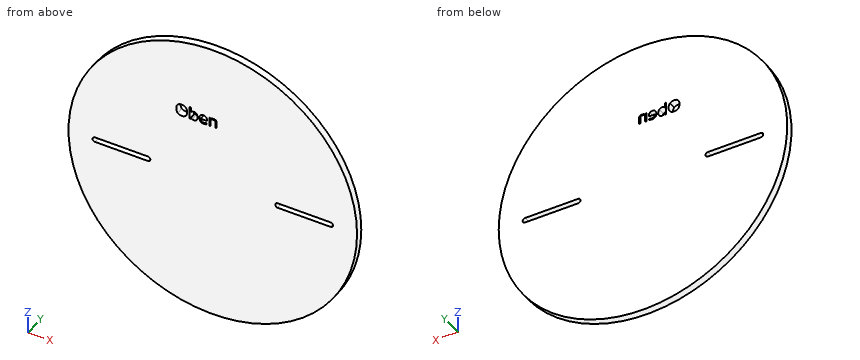
from build123d import *

# Parameters (mm, degrees)
F0_R     = 300.0001975894
F1_DEPTH = 15


with BuildPart() as f1:
    # F0 (on Front) → F1 (new body)
    with BuildSketch(Plane.XZ):
        Circle(F0_R)
        with BuildLine():
            ThreePointArc((-245.0001975894, -5.1), (-250.1001975894, 0), (-245.0001975894, 5.1))
            Line((-245.0001975894, 5.1), (-135, 5.1))
            ThreePointArc((-135, 5.1), (-129.9, 0), (-135, -5.1))
            Line((-135, -5.1), (-245.0001975894, -5.1))
        make_face(mode=Mode.SUBTRACT)
        with BuildLine():
            ThreePointArc((135.0291466713, -5.1012321273), (129.9, -0.0303787986), (134.9708533287, 5.0987678727))
            Line((134.9708533287, 5.0987678727), (245.0001975894, 5.0987678727))
            ThreePointArc((245.0001975894, 5.0987678727), (250.1001975894, -0.0012321273), (245.0001975894, -5.1012321273))
            Line((245.0001975894, -5.1012321273), (135.0291466713, -5.1012321273))
        make_face(mode=Mode.SUBTRACT)
        with BuildLine():
            add(Edge.make_bspline(
                [(-56.2059473305, 147.280047389), (-53.2054559961, 143.8888953384), (-53.2054559961, 137.9204677295)],
                knots=[0, 0, 0, 1, 1, 1], degree=2))
            add(Edge.make_bspline(
                [(-53.2054559961, 137.9204677295), (-53.2054559961, 131.9683176504), (-56.216799017, 128.5581751484)],
                knots=[0, 0, 0, 1, 1, 1], degree=2))
            add(Edge.make_bspline(
                [(-56.216799017, 128.5581751484), (-59.2281420379, 125.1480326464), (-64.5834493561, 125.1480326464)],
                knots=[0, 0, 0, 1, 1, 1], degree=2))
            add(Edge.make_bspline(
                [(-64.5834493561, 125.1480326464), (-70.0581252264, 125.1480326464), (-73.034200266, 128.4984908723)],
                knots=[0, 0, 0, 1, 1, 1], degree=2))
            add(Edge.make_bspline(
                [(-73.034200266, 128.4984908723), (-76.0102753055, 131.8489490982), (-76.0102753055, 137.9530227892)],
                knots=[0, 0, 0, 1, 1, 1], degree=2))
            add(Edge.make_bspline(
                [(-76.0102753055, 137.9530227892), (-76.0102753055, 144.0082638906), (-73.0260615011, 147.339731665)],
                knots=[0, 0, 0, 1, 1, 1], degree=2))
            add(Edge.make_bspline(
                [(-73.0260615011, 147.339731665), (-70.0418476966, 150.6711994395), (-64.5508942964, 150.6711994395)],
                knots=[0, 0, 0, 1, 1, 1], degree=2))
            add(Edge.make_bspline(
                [(-64.5508942964, 150.6711994395), (-59.2064386648, 150.6711994395), (-56.2059473305, 147.280047389)],
                knots=[0, 0, 0, 1, 1, 1], degree=2))
        make_face(mode=Mode.SUBTRACT)
        with BuildLine():
            add(Edge.make_bspline(
                [(-45.2891506494, 141.5991894739), (-43.3249953817, 144.3772212337), (-39.4563691225, 144.3772212337)],
                knots=[0, 0, 0, 1, 1, 1], degree=2))
            add(Edge.make_bspline(
                [(-39.4563691225, 144.3772212337), (-35.7939249079, 144.3772212337), (-33.7673724425, 141.8759074812)],
                knots=[0, 0, 0, 1, 1, 1], degree=2))
            add(Edge.make_bspline(
                [(-33.7673724425, 141.8759074812), (-31.7408199771, 139.3745937288), (-31.7408199771, 134.800607843)],
                knots=[0, 0, 0, 1, 1, 1], degree=2))
            add(Edge.make_bspline(
                [(-31.7408199771, 134.800607843), (-31.7408199771, 130.221196114), (-33.7836499724, 127.6846143802)],
                knots=[0, 0, 0, 1, 1, 1], degree=2))
            add(Edge.make_bspline(
                [(-33.7836499724, 127.6846143802), (-35.8264799676, 125.1480326464), (-39.4563691225, 125.1480326464)],
                knots=[0, 0, 0, 1, 1, 1], degree=2))
            add(Edge.make_bspline(
                [(-39.4563691225, 125.1480326464), (-41.2740266216, 125.1480326464), (-42.7742722887, 125.8181242916)],
                knots=[0, 0, 0, 1, 1, 1], degree=2))
            add(Edge.make_bspline(
                [(-42.7742722887, 125.8181242916), (-44.2745179559, 126.4882159368), (-45.2891506494, 127.8826576599)],
                knots=[0, 0, 0, 1, 1, 1], degree=2))
            Line((-45.2891506494, 127.8826576599), (-45.4953326941, 127.8826576599))
            Line((-45.4953326941, 127.8826576599), (-46.0867496117, 125.4898607731))
            Line((-46.0867496117, 125.4898607731), (-48.1051633122, 125.4898607731))
            Line((-48.1051633122, 125.4898607731), (-48.1051633122, 151.8757366478))
            Line((-48.1051633122, 151.8757366478), (-45.2891506494, 151.8757366478))
            Line((-45.2891506494, 151.8757366478), (-45.2891506494, 145.4623898899))
            add(Edge.make_bspline(
                [(-45.2891506494, 145.4623898899), (-45.2891506494, 143.3083301074), (-45.4247967314, 141.5991894739)],
                knots=[0, 0, 0, 1, 1, 1], degree=2))
            Line((-45.4247967314, 141.5991894739), (-45.2891506494, 141.5991894739))
        make_face(mode=Mode.SUBTRACT)
        with BuildLine():
            add(Edge.make_bspline(
                [(-15.761711515, 125.430176497), (-17.0910431189, 125.1480326464), (-18.9738107373, 125.1480326464)],
                knots=[0, 0, 0, 1, 1, 1], degree=2))
            add(Edge.make_bspline(
                [(-18.9738107373, 125.1480326464), (-23.0920257875, 125.1480326464), (-25.4766839094, 127.6601980854)],
                knots=[0, 0, 0, 1, 1, 1], degree=2))
            add(Edge.make_bspline(
                [(-25.4766839094, 127.6601980854), (-27.8613420313, 130.1723635245), (-27.8613420313, 134.626980858)],
                knots=[0, 0, 0, 1, 1, 1], degree=2))
            add(Edge.make_bspline(
                [(-27.8613420313, 134.626980858), (-27.8613420313, 139.1250049378), (-25.6475979727, 141.7701035373)],
                knots=[0, 0, 0, 1, 1, 1], degree=2))
            add(Edge.make_bspline(
                [(-25.6475979727, 141.7701035373), (-23.4338539142, 144.4152021367), (-19.7008737369, 144.4152021367)],
                knots=[0, 0, 0, 1, 1, 1], degree=2))
            add(Edge.make_bspline(
                [(-19.7008737369, 144.4152021367), (-16.2120565074, 144.4152021367), (-14.177365277, 142.1173575072)],
                knots=[0, 0, 0, 1, 1, 1], degree=2))
            add(Edge.make_bspline(
                [(-14.177365277, 142.1173575072), (-12.1426740467, 139.8195128778), (-12.1426740467, 136.0539776409)],
                knots=[0, 0, 0, 1, 1, 1], degree=2))
            Line((-12.1426740467, 136.0539776409), (-12.1426740467, 134.2743010448))
            Line((-12.1426740467, 134.2743010448), (-24.9422383462, 134.2743010448))
            add(Edge.make_bspline(
                [(-24.9422383462, 134.2743010448), (-24.8554248537, 131.0025175464), (-23.2873561456, 129.3069415212)],
                knots=[0, 0, 0, 1, 1, 1], degree=2))
            add(Edge.make_bspline(
                [(-23.2873561456, 129.3069415212), (-21.7192874374, 127.6113654959), (-18.870719715, 127.6113654959)],
                knots=[0, 0, 0, 1, 1, 1], degree=2))
            add(Edge.make_bspline(
                [(-18.870719715, 127.6113654959), (-15.8702283807, 127.6113654959), (-12.940273009, 128.8647352938)],
                knots=[0, 0, 0, 1, 1, 1], degree=2))
            Line((-12.940273009, 128.8647352938), (-12.940273009, 126.3525698547))
            add(Edge.make_bspline(
                [(-12.940273009, 126.3525698547), (-14.4323799112, 125.7123203476), (-15.761711515, 125.430176497)],
                knots=[0, 0, 0, 1, 1, 1], degree=2))
        make_face(mode=Mode.SUBTRACT)
        with BuildLine():
            Line((8.1933865699, 125.4898607731), (5.3773739071, 125.4898607731))
            Line((5.3773739071, 125.4898607731), (5.3773739071, 137.5135294834))
            add(Edge.make_bspline(
                [(5.3773739071, 137.5135294834), (5.3773739071, 139.7815319748), (4.3437507621, 140.9019686123)],
                knots=[0, 0, 0, 1, 1, 1], degree=2))
            add(Edge.make_bspline(
                [(4.3437507621, 140.9019686123), (3.3101276171, 142.0224052498), (1.1018094018, 142.0224052498)],
                knots=[0, 0, 0, 1, 1, 1], degree=2))
            add(Edge.make_bspline(
                [(1.1018094018, 142.0224052498), (-1.81186844, 142.0224052498), (-3.1683292602, 140.4461977767)],
                knots=[0, 0, 0, 1, 1, 1], degree=2))
            add(Edge.make_bspline(
                [(-3.1683292602, 140.4461977767), (-4.5247900804, 138.8699903036), (-4.5247900804, 135.2401011488)],
                knots=[0, 0, 0, 1, 1, 1], degree=2))
            Line((-4.5247900804, 135.2401011488), (-4.5247900804, 125.4898607731))
            Line((-4.5247900804, 125.4898607731), (-7.3408027432, 125.4898607731))
            Line((-7.3408027432, 125.4898607731), (-7.3408027432, 144.07337401))
            Line((-7.3408027432, 144.07337401), (-5.0510968787, 144.07337401))
            Line((-5.0510968787, 144.07337401), (-4.5953260431, 141.5286535113))
            Line((-4.5953260431, 141.5286535113), (-4.459679961, 141.5286535113))
            add(Edge.make_bspline(
                [(-4.459679961, 141.5286535113), (-3.5915450361, 142.9013918613), (-2.0316150929, 143.658296999)],
                knots=[0, 0, 0, 1, 1, 1], degree=2))
            add(Edge.make_bspline(
                [(-2.0316150929, 143.658296999), (-0.4716851496, 144.4152021367), (1.4436375285, 144.4152021367)],
                knots=[0, 0, 0, 1, 1, 1], degree=2))
            add(Edge.make_bspline(
                [(1.4436375285, 144.4152021367), (4.8022345194, 144.4152021367), (6.4978105446, 142.7955879173)],
                knots=[0, 0, 0, 1, 1, 1], degree=2))
            add(Edge.make_bspline(
                [(6.4978105446, 142.7955879173), (8.1933865699, 141.175973698), (8.1933865699, 137.6111946625)],
                knots=[0, 0, 0, 1, 1, 1], degree=2))
            Line((8.1933865699, 137.6111946625), (8.1933865699, 125.4898607731))
        make_face(mode=Mode.SUBTRACT)
    extrude(amount=F1_DEPTH)


solid = f1.part
The model under review builds one solid part; all positions refer to its coordinate system, in mm. Round coordinates to 2 decimals unless told otherwise and drop trailing zeros. Loops run counter-clockwise (first coordinate to the right, second up) from the corner with the lowest first, then second, coordinate; pieces in that order, holes last. Notation, with made-up numbers: M -14,66.5 L 6,66.5 A28 ccw 6,95.5 Z; hole C 62,-4 d6. An arc over 180 degrees is marked long. Answer as a JSON object with one key per item and string values.
Item 1: We need section C-C, the plane z = -175. State the section outline as (x, y) points.
Check sheet entries:
{"outline": "M -243.67,-15 L 243.67,-15 L 243.67,0 L -243.67,0 Z"}
Item 2: We need section D-D, the plane x = -192. State the section outline as (y, z) points.
Check sheet entries:
{"outline": "M -15,-230.51 L 0,-230.51 L 0,-5.1 L -15,-5.1 Z; M -15,5.1 L 0,5.1 L 0,230.51 L -15,230.51 Z"}
Item 3: We need section B-B, the plane y = -3.5. State how many separate pieces and enclosed holes the cut face has, and give its area (3 significant figures).
Check sheet entries:
{"separate pieces": "1", "enclosed holes": "6", "area": "279,000 mm2"}
Item 4: We need section A-A, the plane x = 169. State the section outline as (y, z) points, and give its area (3 significant figures).
Check sheet entries:
{"outline": "M -15,-247.87 L 0,-247.87 L 0,-5.1 L -15,-5.1 Z; M -15,5.1 L 0,5.1 L 0,247.87 L -15,247.87 Z", "area": "7,280 mm2"}
Item 5: Clearance check with flat-ended pins moving along their axes: P1, Ø1.4, axis at x = -6, y = -4, coming from the +Z side; P2, Ø1, axis at x = -128, y = -13, coming from the +Z side; P3, Ø2.5, axis at x = -46, y = -5.5, coming from the -Z side. State where each tip first meets the part, or that it passes through.
Check sheet entries:
{"P1": "z = 299.95", "P2": "z = 271.56", "P3": "z = -296.64"}
Item 6: For line 1 along Z through (x, y) = (-40.5, -8.5); line 2 along Z through (x, y) = (-144.5, -10.25); line 3 along X through (y, z) = (-7.5, -116), list the stretches that pass through material, from the lowest coordinate up.
Check sheet entries:
{"line 1": "-297.25 to 125.21, 144.32 to 297.25", "line 2": "-262.91 to -5.1, 5.1 to 262.91", "line 3": "-276.67 to 276.67"}
